from build123d import *

# Parameters (mm, degrees)
SKETCH1_W           = 198.12
SKETCH1_H           = 247.65
BOSS_EXTRUDE1_DEPTH = 3.175
CUT_EXTRUDE1_REACH  = 5.175
FILLET1_R           = 3.175


with BuildPart() as part:
    # Sketch1 → Boss-Extrude1 (new body)
    with BuildSketch(Plane.XY):
        Rectangle(SKETCH1_W, SKETCH1_H)
    extrude(amount=BOSS_EXTRUDE1_DEPTH)

    # Sketch2 → Cut-Extrude1 (cut, up to next)
    with BuildSketch(Plane.XY.offset(3.175), mode=Mode.PRIVATE) as cut_extrude1_sk1:
        Polygon((-80.01, -87.393535256), (-12.065, 0), (-80.01, 87.393535256), align=None)
    cut_extrude1_tool1 = extrude(cut_extrude1_sk1.sketch, amount=-CUT_EXTRUDE1_REACH, mode=Mode.PRIVATE) & part.part
    add(cut_extrude1_tool1.solids().sort_by_distance((-57.361667, 0, 3.175))[0], mode=Mode.SUBTRACT)
    # Sketch2 → Cut-Extrude1 (cut, up to next)
    with BuildSketch(Plane.XY.offset(3.175), mode=Mode.PRIVATE) as cut_extrude1_sk2:
        Polygon((69.393397971, 104.775), (-69.393397971, 104.775), (0, 15.518478223), align=None)
    cut_extrude1_tool2 = extrude(cut_extrude1_sk2.sketch, amount=-CUT_EXTRUDE1_REACH, mode=Mode.PRIVATE) & part.part
    add(cut_extrude1_tool2.solids().sort_by_distance((0, 75.022826, 3.175))[0], mode=Mode.SUBTRACT)
    # Sketch2 → Cut-Extrude1 (cut, up to next)
    with BuildSketch(Plane.XY.offset(3.175), mode=Mode.PRIVATE) as cut_extrude1_sk3:
        Polygon((80.01, 87.393535256), (12.065, 0), (80.01, -87.393535256), align=None)
    cut_extrude1_tool3 = extrude(cut_extrude1_sk3.sketch, amount=-CUT_EXTRUDE1_REACH, mode=Mode.PRIVATE) & part.part
    add(cut_extrude1_tool3.solids().sort_by_distance((57.361667, 0, 3.175))[0], mode=Mode.SUBTRACT)
    # Sketch2 → Cut-Extrude1 (cut, up to next)
    with BuildSketch(Plane.XY.offset(3.175), mode=Mode.PRIVATE) as cut_extrude1_sk4:
        Polygon((69.393397971, -104.775), (0, -15.518478223), (-69.393397971, -104.775), align=None)
    cut_extrude1_tool4 = extrude(cut_extrude1_sk4.sketch, amount=-CUT_EXTRUDE1_REACH, mode=Mode.PRIVATE) & part.part
    add(cut_extrude1_tool4.solids().sort_by_distance((0, -75.022826, 3.175))[0], mode=Mode.SUBTRACT)

    # Fillet1
    fillet1_edges = [part.edges().sort_by_distance(p)[0] for p in [
        (12.065, 0, 1.5875),
        (80.01, 87.393535256, 1.5875),
        (80.01, -87.393535256, 1.5875),
        (0, 15.518478223, 1.5875),
        (-69.393397971, 104.775, 1.5875),
        (69.393397971, 104.775, 1.5875),
        (-69.393397971, -104.775, 1.5875),
        (0, -15.518478223, 1.5875),
        (69.393397971, -104.775, 1.5875),
        (-80.01, -87.393535256, 1.5875),
        (-80.01, 87.393535256, 1.5875),
        (-12.065, 0, 1.5875),
    ]]
    fillet(fillet1_edges, radius=FILLET1_R)


solid = part.part
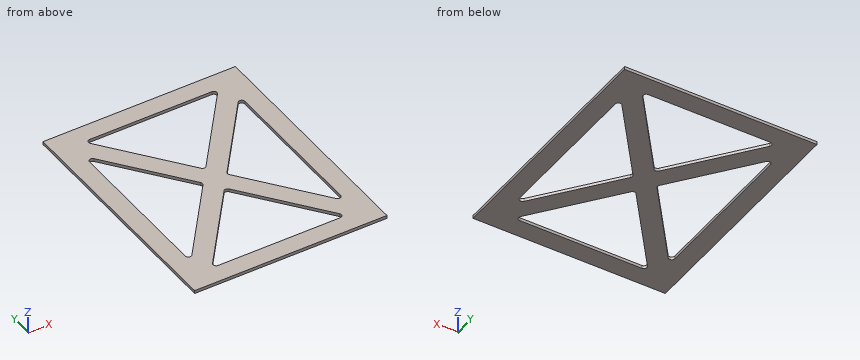
The listing builds one solid part. Answer for the finished solid, in the listing's coordinates (mm). Round coordinates to 2 decimals unless told otherwise and drop trailing zeros. Order: outer loops, then holes, each group sorted by start corner. A loop starts at its lowest first (then second) coordinate and runs counter-clockwise, first axis right, second up. Notation, with made-up numbers: M 25.25,22.5 L 72.25,22.5 A14 cw 72.25,28.5 Z; hole C 49,20 d9. An arc over 180 degrees is marked long. Answer in a Markdown table with one row per item. Add a question column.
1) The part is cut by section C-C on x = -28.5. Determine the outline of the cut face in (y, z) (3 decimals), plus the area to 3 significant figures.
2) A flat-ended cylindrical pin translates along its axis: pin 1 Ø5 at (x, y) = (-58, -96.5) entering from +Z. Find the tip coordinate at first contact, or state that the pin passes through.
3) The part is cut by section B-B on y = 45.5. Determine the outline of the cut face in (x, z) (3 decimals).
4) The part is cut by section A-A on z = 1.85. Determine the outline of the cut face in (x, y) (3 decimals), plus the area to 3 significant figures.
5) Consider line 1 along X through (y, z) = (-7, 2.45); line 2 along X through (y, z) = (59, 2.65); line 3 along Y through (x, z) = (47.5, 1.95) (3 decimals). Determine where each line is inside the solid, lowest interval first. Write a range as from..to.
Findings below:
| question | item | result |
|---|---|---|
| 1 | outline | M -123.825,0 L -104.775,0 L -104.775,3.175 L -123.825,3.175 Z; M -52.176,0 L -21.139,0 L -21.139,3.175 L -52.176,3.175 Z; M 21.139,0 L 52.176,0 L 52.176,3.175 L 21.139,3.175 Z; M 104.775,0 L 123.825,0 L 123.825,3.175 L 104.775,3.175 Z |
| 1 | area | 318 mm² |
| 2 | pin 1 | passes through |
| 3 | outline | M -99.06,0 L -80.01,0 L -80.01,3.175 L -99.06,3.175 Z; M -47.439,0 L -23.309,0 L -23.309,3.175 L -47.439,3.175 Z; M 23.309,0 L 47.439,0 L 47.439,3.175 L 23.309,3.175 Z; M 80.01,0 L 99.06,0 L 99.06,3.175 L 80.01,3.175 Z |
| 4 | outline | M -99.06,-123.825 L 99.06,-123.825 L 99.06,123.825 L -99.06,123.825 Z; hole M -80.01,-78.137 A3.175 ccw -74.328,-80.086 L -13.58,-1.949 A3.175 ccw -13.58,1.949 L -74.328,80.086 A3.175 ccw -80.01,78.137 Z; hole M -65.41,-99.651 A3.175 ccw -62.903,-104.775 L 62.903,-104.775 A3.175 ccw 65.41,-99.651 L 2.507,-18.743 A3.175 ccw -2.507,-18.743 Z; hole M -65.41,99.651 L -2.507,18.743 A3.175 ccw 2.507,18.743 L 65.41,99.651 A3.175 ccw 62.903,104.775 L -62.903,104.775 A3.175 ccw Z; hole M 13.58,-1.949 L 74.328,-80.086 A3.175 ccw 80.01,-78.137 L 80.01,78.137 A3.175 ccw 74.328,80.086 L 13.58,1.949 A3.175 ccw Z |
| 4 | area | 24,900 mm² |
| 5 | line 1 | x = -99.06..-80.01, -17.51..17.51, 80.01..99.06 |
| 5 | line 2 | x = -99.06..-80.01, -57.94..-33.81, 33.81..57.94, 80.01..99.06 |
| 5 | line 3 | y = -123.825..-104.775, -76.615..-45.578, 45.578..76.615, 104.775..123.825 |
